Geometry: final body of the model. Coordinates: model frame, mm. Face numbers are marked on the shaded views. A direction names the side the tool comes from. Round coordinates to 2 decimals unless told otherwise and drop trailing zeros. Order: outer loops, then holes, each group sorted by start corner. A loop starts at its lowest first (then second) coordinate and runs counter-clockwise, first axis right, second up. Notation, with made-up numbers: (-21.75, 67.5) -> (-16.75, 67.5) arc R28 cw to (-16.75, 90.5) -> close; hole circle Ø5 at (49, 54.5). An arc over 180 degrees is marked (long way). Put each result on its own line as item: value.
```python
from build123d import *

# Parameters (mm, degrees)
SKETCH_1_W      = 100
SKETCH_1_H      = 50
EXTRUDE_1_DEPTH = 1
SKETCH_2_W      = 17
SKETCH_2_H      = 10
EXTRUDE_2_DEPTH = 6
HOLE_WIZARD_1_D = 3


with BuildPart() as part:
    # 草图1 → 凸台-拉伸1 (new body)
    with BuildSketch(Plane(origin=(0, 0, 0), x_dir=(1, 0, 0), z_dir=(0, 1, 0))):
        Rectangle(SKETCH_1_W, SKETCH_1_H)
    extrude(amount=EXTRUDE_1_DEPTH)

    # 草图2 → 凸台-拉伸2 (add)
    with BuildSketch(Plane(origin=(0, 1, 0), x_dir=(1, 0, 0), z_dir=(0, 1, 0))):
        with Locations((50, 0)):
            Rectangle(SKETCH_2_W, SKETCH_2_H)
    extrude(amount=EXTRUDE_2_DEPTH)

    # 孔1 (through all)
    with Locations(Plane(origin=(0, 1, 0), x_dir=(1, 0, 0), z_dir=(0, 1, 0))):
        with Locations((-44, 20.75), (-44, -20.75), (44, -20.75), (44, 20.75)):
            Hole(HOLE_WIZARD_1_D / 2)


solid = part.part
```
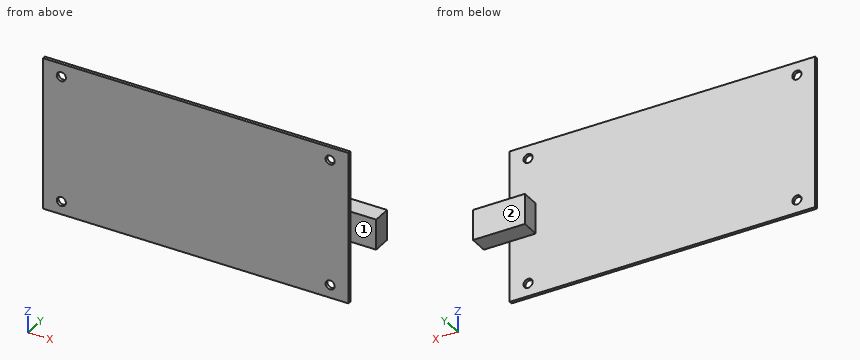
1. Set-up query: the marked faces 1 and 2. Return all of +Z, -Z, +X, -X, +Y, -Y with unobstructed straight access to the full face (end or side cutting, diameter ignored); none if empty.
Ans:
face 1: +Z, -Z, +X, -Y
face 2: +Z, -Z, +X, -X, +Y
2. Cut plane B-B on z = 20.75. Return loops of the section in (x, y), and give its area (3 significant figures).
Ans:
outline: (-50, 0) -> (-45.5, 0) -> (-45.5, 1) -> (-50, 1) -> close; (-42.5, 0) -> (42.5, 0) -> (42.5, 1) -> (-42.5, 1) -> close; (45.5, 0) -> (50, 0) -> (50, 1) -> (45.5, 1) -> close
area: 94.0 mm²
3. Contact query for flat-ended pins moving along their axis: P1, Ø0.5, axis at y = 0.5, z = 6, coming from the +X side; P2, Ø1, axis at x = 1, z = 7.5, coming from the +Y side; P3, Ø1.8, axis at x = 50, y = 4.5, coming from the +Z side. Output: stop coordinate, or through.
Ans:
P1: x = 50
P2: y = 1
P3: z = 5
4. Cut plane A-A on x = 44. Return loops of the section in (y, z), and give its area (3 significant figures).
Ans:
outline: (0, -25) -> (1, -25) -> (1, -22.25) -> (0, -22.25) -> close; (0, -19.25) -> (1, -19.25) -> (1, -5) -> (7, -5) -> (7, 5) -> (1, 5) -> (1, 19.25) -> (0, 19.25) -> close; (0, 22.25) -> (1, 22.25) -> (1, 25) -> (0, 25) -> close
area: 104 mm²
5. Material intervals for probe 1 along Z at (x, y) = (44, 0.4); probe 2 along X at (y, z) = (0.6, 20.75); probe 3 along Y at (x, z) = (33, 14.5), sorted ascending.
Ans:
probe 1: -25 to -22.25, -19.25 to 19.25, 22.25 to 25
probe 2: -50 to -45.5, -42.5 to 42.5, 45.5 to 50
probe 3: 0 to 1
6. Cut plane D-D on y = 5.5. Return loops of the section in (x, z), and give its area (3 significant figures).
Ans:
outline: (41.5, -5) -> (58.5, -5) -> (58.5, 5) -> (41.5, 5) -> close
area: 170 mm²
7. Cut plane C-C on z = 0. Return loops of the section in (x, y).
Ans:
outline: (-50, 0) -> (50, 0) -> (50, 1) -> (58.5, 1) -> (58.5, 7) -> (41.5, 7) -> (41.5, 1) -> (-50, 1) -> close
